Here's how the part is built. I have some questions about the finished solid (model axes, mm). A direction names the side the tool comes from. Round coordinates to 2 decimals unless told otherwise and drop trailing zeros. Loops run counter-clockwise (first coordinate to the right, second up) from the corner with the lowest first, then second, coordinate; pieces in that order, holes last. Notation, with made-up numbers: (75.25, 81.25) -> (103.25, 81.25) arc R20 cw to (103.25, 110.25) -> close; hole circle Ø11 at (66, 83). An arc over 180 degrees is marked (long way). One line per item, written item: value. Start each with the question number.
Autodesk Inventor part; units mm, degrees
ref_plane "YZ Plane" through (0, 0, 0) normal (1, 0, 0) x (0, 1, 0)
ref_plane "XZ Plane" through (0, 0, 0) normal (0, 1, 0) x (-1, 0, 0)
ref_plane "XY Plane" through (0, 0, 0) normal (0, 0, 1) x (1, 0, 0)
sketch "Sketch1" plane through (0, 0, 0) normal (0, 0, 1) x (1, 0, 0)
  line L0 (-12.7, -12.7) -> (12.7, -12.7)
  line L1 (12.7, -12.7) -> (12.7, 12.7)
  line L2 (12.7, 12.7) -> (-12.7, 12.7)
  line L3 (-12.7, 12.7) -> (-12.7, -12.7)
  line L4 (-12.7, -12.7) -> (12.7, 12.7) construction
  line L5 (12.7, -12.7) -> (-12.7, 12.7) construction
  line L6 (-9.525, 9.525) -> (9.525, 9.525)
  line L7 (9.525, 9.525) -> (9.525, -9.525)
  line L8 (9.525, -9.525) -> (-9.525, -9.525)
  line L9 (-9.525, -9.525) -> (-9.525, 9.525)
  point P0 (0, 0)
  dimension "width" = 25.4
  dimension "height" = 25.4
  dimension "thickness" = 3.175
extrude "Extrusion1" add sketch "Sketch1" along normal mid plane 76.2
sketch "Sketch3" plane through (12.7, -12.7, 38.1) normal (1, 0, 0) x (0, 0, -1)
  line L0 (7.9502, 12.7) -> (42.8752, 12.7) construction
  line L1 (0, 0) -> (0, 25.4)
  point P0 (25.4127, 12.7)
  point P1 (0, 12.7)
  dimension "d22" = 34.925
  dimension "d37" = 7.9502
hole "Hole2" at (12.7, 0, -4.7752) at (12.7, 0, 30.1498) direction (-1, 0, 0) diameter 5.1054 end through all
sketch "Sketch4" plane through (-12.7, 12.7, 38.1) normal (0, 1, 0) x (1, 0, 0)
  line L0 (0, 76.2) -> (25.4, 76.2)
  line L1 (0, 76.2) -> (0, 0) construction
  point P0 (12.7, 38.1)
  point P1 (7.62, 65.0875)
  dimension "d38" = 11.1125
  dimension "d39" = 7.62
hole "Hole3" at (-5.08, 12.7, -26.9875) direction (0, -1, 0) diameter 6.7564 end through all
properties part number "EL2-S-004" material "Aluminum 6061"
Q1. I want a section at C-C on z = 26. Please give me the cut outline in (x, y) (3 decimals).
Q2. Which directions (+Z, -Z, +X, -X, +Y, -Y) give clear straight access to the entire face, cutting with the end or side of a thin tool? Please do faces 5 (the flat face through (9.525, 0, -1)), 6 (the flat face through (0, 12.7, -1)).
Q3. I want a section at B-B on x = -5.08. Please give me the cut outline in (y, z) (3 decimals), plus the area to 3 significant figures.
Q4. I want a section at A-A on y = -6.5. Please give me the cut outline in (x, z) (3 decimals).
Q5. If I drill on line 1 along Z through (x, y) = (10.2, 0); line 2 along Y through (x, z) = (-1.25, -3) (3 decimals), over which ranges is the centre line in solid material (lowest first)?
Q6. Will these pins go through, and if not, where does the flat tip stop? P1, Ø4, axis at y = 0, z = 30.15, coming from the -X side; P2, Ø9, axis at x = -5.08, z = -26.99, coming from the +Y side.
Q7. If we mould it in two halves opening along X, with no side actions, what happens to faces 1 (the cylindrical face through (-3.786, -11.135, -23.867)), 2 (the flat face through (12.7, 0, -1)), 3 (the flat face through (11, 0, -38.1)), 4 (the flat face through (0, 9.525, -1))? For each: released by +X, released by -X, zero draft, split by the parting line, or undercut.
Answers below:
1. outline: (-12.7, -12.7) -> (12.7, -12.7) -> (12.7, 12.7) -> (-12.7, 12.7) -> close; hole (-9.525, -9.525) -> (9.525, -9.525) -> (9.525, 9.525) -> (-9.525, 9.525) -> close
2. face 5: +Z, -Z
2. face 6: +Z, -Z, +X, -X, +Y
3. outline: (-12.7, -38.1) -> (-9.525, -38.1) -> (-9.525, -30.366) -> (-12.7, -30.366) -> close; (-12.7, -23.609) -> (-9.525, -23.609) -> (-9.525, 38.1) -> (-12.7, 38.1) -> close; (9.525, -38.1) -> (12.7, -38.1) -> (12.7, -30.366) -> (9.525, -30.366) -> close; (9.525, -23.609) -> (12.7, -23.609) -> (12.7, 38.1) -> (9.525, 38.1) -> close
3. area: 441 mm^2
4. outline: (-12.7, -38.1) -> (-9.525, -38.1) -> (-9.525, 38.1) -> (-12.7, 38.1) -> close; (9.525, -38.1) -> (12.7, -38.1) -> (12.7, 38.1) -> (9.525, 38.1) -> close
5. line 1: z = -38.1 to -7.33, -2.22 to 27.6, 32.7 to 38.1
5. line 2: y = -12.7 to -9.525, 9.525 to 12.7
6. P1: passes through
6. P2: stops at y = 12.7
7. face 1: undercut
7. face 2: released by +X
7. face 3: zero draft
7. face 4: undercut
